Design review of the part built by this model. Coordinates are the model's own, in mm. A direction names the side the tool comes from. Round coordinates to 2 decimals unless told otherwise and drop trailing zeros. Order: outer loops, then holes, each group sorted by start corner. A loop starts at its lowest first (then second) coordinate and runs counter-clockwise, first axis right, second up. Notation, with made-up numbers: M 51.5,33.5 L 57.5,33.5 A14 cw 57.5,49.5 Z; hole C 43.25,-5 d4. An arc over 180 degrees is marked long. Use a Markdown table: item, result. Add a question column.
(1) For pin 1 (2 mm diameter, centred on y = 29, z = 14.5, fed in from -X); pin 2 (3 mm diameter, centred on x = -26.5, z = 18, fed in from -Y); pin 3 (4.5 mm diameter, centred on y = 41.36, z = 8, fed in from +X); pin 4 (3 mm diameter, centred on y = -15.5, z = 47.5, fed in from +X), all flat-tipped, find the tip position at first contact; note any pin that passes through.
(2) To check wall thickness, follow probe 1 along Z at (x, y) = (-24.5, 47); probe 2 along Z at (x, y) = (0.5, 9); probe 3 along Y at (x, z) = (-44.5, -8). State the ranges of each line that lie inside material, in increasing order. Write a range as from..to.
(3) Take a section at B-B (z = 8). Count the separate pieces of the cut face and the enclosed holes in it, then the cut area to 3 significant figures.
(4) The part is to be moulded in two halves that separate along Y. For faces 1 (the face through (0, 1, 60)), 2 (the face through (-14, -8, 49)), 3 (the face through (-41, 52.5, 4)), say which applies: released by +Y, released by -Y, zero draft, split by the parting line, or undercut.
(5) Machinability: for faces 4 (the face through (-48.817, 44.827, -8.456)), 5 (the face through (-27.815, 39.139, 42.255)), 6 (the face through (0, 2.5, 0)), 7 (the face through (-14, -8, -49)), which of the approach directions +Z, -Z, +X, -X, +Y, -Y give a long, thin tool a straight path to every point of the face, cutting with its end or side? Answer none if there is none.
(6) Take a section at A-A (x = -2). Write out the cut boundary in (y, z), then the cut area to 3 significant figures.
```python
from build123d import *

# Parameters (mm, degrees)
CROQUIS1_R                                           = 2.5
SALIENTE_EXTRUIR1_DEPTH                              = 5
CROQUIS9_W                                           = 90
CROQUIS9_H                                           = 55
SALIENTE_EXTRUIR2_DEPTH                              = 10
REFRENTADO_PARA_TORNILLO_CON_CABEZA_TRON_D           = 3.4
REFRENTADO_PARA_TORNILLO_CON_CABEZA_TRON_DEPTH       = 10
REFRENTADO_PARA_TORNILLO_CON_CABEZA_TRON_CBORE_D     = 7
REFRENTADO_PARA_TORNILLO_CON_CABEZA_TRON_CBORE_DEPTH = 2.4
CORTAR_EXTRUIR1_DEPTH                                = 45


with BuildPart() as part:
    # Croquis1 → Saliente-Extruir1 (new, symmetric)
    with BuildSketch(Plane(origin=(0, 0, 0), x_dir=(0, 0, -1), z_dir=(1, 0, 0))):
        Polygon((-60, 52.5), (-60, -52.5), (60, -52.5), (60, 52.5), (30, 52.5), (30, 2.5), (-30, 2.5), (-30, 52.5), align=None)
        with Locations((-47.5, -15.5)):
            Circle(CROQUIS1_R, mode=Mode.SUBTRACT)
        with Locations((47.5, -15.5)):
            Circle(CROQUIS1_R, mode=Mode.SUBTRACT)
        with Locations((-47.5, 44.5)):
            Circle(CROQUIS1_R, mode=Mode.SUBTRACT)
        with Locations((47.5, 44.5)):
            Circle(CROQUIS1_R, mode=Mode.SUBTRACT)
    extrude(amount=SALIENTE_EXTRUIR1_DEPTH, both=True)

    # Croquis7 → Recubrir3 section 0
    with BuildSketch(Plane.ZY.offset(5)):
        with BuildLine():
            Line((-52.5, -42.5), (52.5, -42.5))
            Line((52.5, -42.5), (52.5, 52.5))
            Line((52.5, 52.5), (35, 52.5))
            Line((35, 52.5), (35, -2.5))
            Line((35, -2.5), (-35, -2.5))
            Line((-35, -2.5), (-35, 52.5))
            Line((-35, 52.5), (-52.5, 52.5))
            Line((-52.5, 52.5), (-52.5, -42.5))
        make_face()
    # Croquis8 → Recubrir3 section 1
    with BuildSketch(Plane(origin=(-50, 0, 0), x_dir=(0, 0, -1), z_dir=(1, 0, 0))):
        with BuildLine():
            Line((-45, -2.5), (45, -2.5))
            Line((45, -2.5), (45, 52.5))
            Line((45, 52.5), (35, 52.5))
            Line((35, 52.5), (35, 7.5))
            Line((35, 7.5), (-35, 7.5))
            Line((-35, 7.5), (-35, 52.5))
            Line((-35, 52.5), (-45, 52.5))
            Line((-45, 52.5), (-45, -2.5))
        make_face()
    loft()

    # Croquis9 → Saliente-Extruir2 (add)
    with BuildSketch(Plane.ZY.offset(50)):
        with Locations((0, 25)):
            Rectangle(CROQUIS9_W, CROQUIS9_H)
    extrude(amount=-SALIENTE_EXTRUIR2_DEPTH)

    # Refrentado para tornillo con cabeza troncocónica de M34
    with Locations(Plane.ZY.offset(50)):
        with Locations((-8, 41.356406461), (8, 41.356406461), (16, 27.5), (8, 13.643593539), (-8, 13.643593539), (-16, 27.5), (-99.109009009, 35.557197268)):
            CounterBoreHole(REFRENTADO_PARA_TORNILLO_CON_CABEZA_TRON_D / 2, REFRENTADO_PARA_TORNILLO_CON_CABEZA_TRON_CBORE_D / 2, REFRENTADO_PARA_TORNILLO_CON_CABEZA_TRON_CBORE_DEPTH, depth=REFRENTADO_PARA_TORNILLO_CON_CABEZA_TRON_DEPTH)

    # Croquis12 → Cortar-Extruir1 (cut)
    with BuildSketch(Plane.ZY.offset(50)):
        with BuildLine():
            Line((-40, 44.5), (-40, 52.5))
            Line((-40, 52.5), (-55, 52.5))
            Line((-55, 52.5), (-55, 44.5))
            Line((-55, 44.5), (-55, 37))
            Line((-55, 37), (-47.5, 37))
            ThreePointArc((-47.5, 37), (-42.196699141, 39.196699141), (-40, 44.5))
        make_face()
        with BuildLine():
            Line((40, 44.5), (40, 52.5))
            Line((40, 52.5), (55, 52.5))
            Line((55, 52.5), (55, 44.5))
            Line((55, 44.5), (55, 37))
            Line((55, 37), (47.5, 37))
            ThreePointArc((47.5, 37), (42.196699141, 39.196699141), (40, 44.5))
        make_face()
        with BuildLine():
            Line((47.5, -8), (55, -8))
            Line((55, -8), (55, -15.5))
            Line((55, -15.5), (55, -23))
            Line((55, -23), (47.5, -23))
            ThreePointArc((47.5, -23), (40, -15.5), (47.5, -8))
        make_face()
        with BuildLine():
            Line((-47.5, -8), (-55, -8))
            Line((-55, -8), (-55, -15.5))
            Line((-55, -15.5), (-55, -23))
            Line((-55, -23), (-47.5, -23))
            ThreePointArc((-47.5, -23), (-40, -15.5), (-47.5, -8))
        make_face()
    extrude(amount=-CORTAR_EXTRUIR1_DEPTH, mode=Mode.SUBTRACT)


solid = part.part
```
Verdict:
| question | item | result |
|---|---|---|
| 1 | pin 1 | stops at x = -47.6 |
| 1 | pin 2 | stops at y = -24.72 |
| 1 | pin 3 | stops at x = -40 |
| 1 | pin 4 | passes through |
| 2 | probe 1 | z = -40..-35, 35..40 |
| 2 | probe 2 | z = -60..-30, 30..60 |
| 2 | probe 3 | y = -7.39..11.94, 15.34..39.66, 43.06..52.5 |
| 3 | separate pieces | 3 |
| 3 | enclosed holes | 0 |
| 3 | area | 2,050 mm^2 |
| 4 | face 1 | zero draft |
| 4 | face 2 | undercut |
| 4 | face 3 | released by +Y |
| 5 | face 4 | -X |
| 5 | face 5 | +Z, -X, +Y |
| 5 | face 6 | +X, +Y |
| 5 | face 7 | -Z, -X |
| 6 | outline | M -52.5,-60 L 52.5,-60 L 52.5,-30 L 2.5,-30 L 2.5,30 L 52.5,30 L 52.5,60 L -52.5,60 Z; hole C -15.5,-47.5 d5; hole C -15.5,47.5 d5; hole C 44.5,-47.5 d5; hole C 44.5,47.5 d5 |
| 6 | area | 9,520 mm^2 |
